The model under review builds one solid part; all positions refer to its coordinate system, in mm. A direction names the side the tool comes from. Round coordinates to 2 decimals unless told otherwise and drop trailing zeros. Order: outer loops, then holes, each group sorted by start corner. A loop starts at its lowest first (then second) coordinate and runs counter-clockwise, first axis right, second up. Notation, with made-up numbers: (23.25, 87) -> (74.25, 87) arc R21 cw to (74.25, 91) -> close; hole circle Ø10 at (10.25, -18.5). An arc over 180 degrees is marked (long way). Put each result on its own line as item: value. Start each with the question number.
Autodesk Inventor part; units mm, degrees
ref_plane "YZ Plane" through (0, 0, 0) normal (1, 0, 0) x (0, 1, 0)
ref_plane "XZ Plane" through (0, 0, 0) normal (0, 1, 0) x (-1, 0, 0)
ref_plane "XY Plane" through (0, 0, 0) normal (0, 0, 1) x (1, 0, 0)
sketch "Sketch4" plane through (0, 0, 0) normal (0, 0, 1) x (1, 0, 0)
  line L0 (-3.1, 0) -> (12, 0)
  line L1 (0, 0) -> (-3.1, 0)
  line L2 (0, 4) -> (0, 2.66)
  line L3 (0.7, 1.96) -> (0.7, 1.96)
  line L4 (0.7, 1.96) -> (1.4, 2)
  arc A0 (0, 2.66) -> (0.7, 1.96) centre (0.7, 2.66) ccw
  line L5 (-3.1, 0) -> (-3.1, 2)
  line L6 (0, 4) -> (-1.5716, 4)
  arc A1 (-1.5716, 4) -> (-3.1, 2) centre (2.731, -0.8721) ccw
  line L7 (1.4, 2) -> (12, 2)
  line L8 (12, 2) -> (12, 0)
  point P0 (0, 1.96)
  dimension "d71" = 0.7
  dimension "d72" = 12
  dimension "d74" = 0.7
  dimension "d75" = 3.92
  dimension "d78" = 4
  dimension "d82" = 6.5
  dimension "d83" = 3.1
  dimension "d84" = 8
  dimension "d104" = 10.6
  dimension "d105" = 4
revolve "Revolution7" add sketch "Sketch4" angle 360 about axis through (-3.1, 0, 0) along (1, 0, 0)
sketch "Sketch5" plane through (-3.1, 0, 0) normal (-1, 0, 0) x (0, 0, 1)
  circle A0 centre (0, 0) radius 1.975 construction
  circle A1 centre (0, 0) radius 1.3825 construction
  line L0 (0, 0) -> (-1.1973, 0.6912)
  line L1 (0, 0) -> (-1.1973, -0.6912)
  line L2 (-1.8008, 0) -> (1.7887, 0)
  line L3 (-1.975, 0) -> (-1.1973, -0.6912)
  line L4 (-1.975, 0) -> (-1.1973, 0.6912)
  point P0 (0, 0)
  dimension "d88" = 3.95
  dimension "d89" = 2.765
  dimension "d90" = 30
  dimension "d91" = 30
extrude "Extrusion1" cut sketch "Sketch5" against normal blind 1.66
pattern_circular "Circular Pattern1" count 6 over 360 about axis through (-10, 0, 0) along (1, 0, 0) of "Extrusion1"
fillet "Fillet1" radius 0.395 12 edges at (-2.27, -1.7104, -0.9875) (-2.27, -0.6912, -1.1973) (-2.27, -1.3825, 0) (-2.27, -1.7104, 0.9875) (-2.27, -0.6912, 1.1973) (-2.27, 0, 1.975) (-2.27, 1.3825, 0) (-2.27, 1.7104, 0.9875) (-2.27, 0.6913, 1.1973) (-2.27, 0.6912, -1.1973) (-2.27, 0, -1.975) (-2.27, 1.7104, -0.9875)
thread "Thread7"
equation "\"a\" = 1.4"
equation "\"b\" = 10.6"
equation "\"dk\" = 8"
equation "\"k\" = 3.1"
equation "\"r\" = 0.7"
equation "\"rf\" = 6.5"
equation "\"x\" = 0.7"
equation "\"A_\" = 3.95"
equation "\"t\" = 1.66"
equation "\"p\" = 0.7"
equation "\"l_\" = 12"
equation "\"d\" = 4"
equation "\"ds_\" = 3.92"
equation "\"lg\" = 0"
properties part number "Flachkopfschraube mit Innenrund ISO 14583 - M4 x 12 - A3-70" material "Edelstahl"
Q1. Wall thickness on probe 1 along X at (y, z) = (0, -1); probe 2 along Z at (x, y) = (-1.75, 3.5); probe 3 along X at (y, z) = (-2, 1.5): over which ranges is each line inside the solid? List them lowest first. Write a range as [from, to].
Q2. Draft analysis for pull direction Z (two halves, no side actions). For faces 1 (the face through (0, 3, -1)), 2 (the face through (-0.797, -0.867, 3.905)), 3 (the face through (-1.44, 0, 0)), state which applies: +Z half, -Z half, draft (parallel to the pull), parting line (faces both ways), or undercut.
Q3. Take a section at A-A on x = -1. Give the boundary of the cut face in (y, z).
Q4. Clearance check with flat-ended pins moving along their axes: pin 1 Ø2 at (x, y) = (8, 2.5) entering from -Z; pin 2 Ø3 at (x, y) = (1, 2) entering from +Z. State where each tip first meets the part, or that it passes through.
Q5. For faces 4 (the face through (7, 0, -2)), 5 (the face through (12, 0, 0)), 6 (the face through (0.977, 1.885, 0.593)), list the 3-axis set-ups (+Z, -Z, +X, -X, +Y, -Y) from which the entire face can be reached by the end or side of a thin tool; tool diameter is ignored.
Q6. Take a section at B-B on x = 9. Give the boundary of the cut face in (y, z), and give its area (3 significant figures).
Calculated:
1. probe 1: x = [-1.44, 12]
1. probe 2: z = [-1.57, 1.57]
1. probe 3: x = [-2.83, 0.02]
2. face 1: draft
2. face 2: parting line
2. face 3: undercut
3. outline: circle Ø8 at (0, 0)
4. pin 1: stops at z = -1.32
4. pin 2: stops at z = 3.9
5. face 4: +X
5. face 5: +Z, -Z, +X, +Y, -Y
5. face 6: none
6. outline: circle Ø4 at (0, 0)
6. area: 12.6 mm²
